Design review of the part built by this model. Coordinates are the model's own, in mm. A direction names the side the tool comes from. Give positions to 0.01 mm unless a question says otherwise; leave off trailing zeros. Loops run counter-clockwise (first coordinate to the right, second up) from the corner with the lowest first, then second, coordinate; pieces in that order, holes last. Notation, with made-up numbers: (55.5, -7.5) -> (103.5, -7.5) arc R29 cw to (103.5, 17.5) -> close; hole circle Ø5 at (65.25, 39.25). An arc over 180 degrees is marked (long way). Answer as CSV lines item,"result".
from build123d import *

# Parameters (mm, degrees)
SKETCH1_W            = 30
SKETCH1_H            = 9
BOSS_EXTRUDE1_DEPTH  = 6
CUT_EXTRUDE1_DEPTH   = 7
LPATTERN2_COUNT      = 8
LPATTERN2_PITCH      = 2
LPATTERN2_COL_COUNT  = 8
LPATTERN2_COL_PITCH  = 2
M3_CLEARANCE_HOLE1_D = 3.2
FILLET1_R            = 5


with BuildPart() as part:
    # Sketch1 → Boss-Extrude1 (new body)
    with BuildSketch(Plane(origin=(0, 0, 0), x_dir=(1, 0, 0), z_dir=(0, 1, 0))):
        with Locations((15, 4.5)):
            Rectangle(SKETCH1_W, SKETCH1_H)
    extrude(amount=BOSS_EXTRUDE1_DEPTH)

    # Sketch2 → Cut-Extrude1 (cut, through all)
    with BuildSketch(Plane(origin=(0, 6, 0), x_dir=(1, 0, 0), z_dir=(0, 1, 0))):
        Polygon((14.41183651, 9), (15.58816349, 9), (15.41183651, 8), (14.58816349, 8), align=None)
    cut_extrude1 = extrude(amount=-CUT_EXTRUDE1_DEPTH, mode=Mode.SUBTRACT)

    # LPattern2: Cut-Extrude1 ×8
    with Locations(*[(-i * LPATTERN2_PITCH, 0, 0) for i in range(1, LPATTERN2_COUNT)]):
        add(cut_extrude1, mode=Mode.SUBTRACT)

    # LPattern2 col: Cut-Extrude1 ×8
    with Locations(*[(i * LPATTERN2_COL_PITCH, 0, 0) for i in range(1, LPATTERN2_COL_COUNT)]):
        add(cut_extrude1, mode=Mode.SUBTRACT)

    # M3 Clearance Hole1 (through all)
    with Locations(Plane(origin=(0, 6, 0), x_dir=(1, 0, 0), z_dir=(0, 1, 0))):
        with Locations((5, 5), (25, 5)):
            Hole(M3_CLEARANCE_HOLE1_D / 2)

    # Fillet1
    fillet1_edges = [part.edges().sort_by_distance(p)[0] for p in [
        (30, 3, 0),
        (0, 3, 0),
    ]]
    fillet(fillet1_edges, radius=FILLET1_R)


solid = part.part
Q1. We need section B-B, the plane z = -3. State the section outline as (x, y) points, and give its area (3 significant figures).
Filled sheet:
outline,"(0.42, 0) -> (29.58, 0) -> (29.58, 6) -> (0.42, 6) -> close"
area,"175 mm^2"
Q2. We need section A-A, the plane y = 4. State how many separate pieces and enclosed holes the cut face has, and give its area (3 significant figures).
Filled sheet:
separate pieces,"1"
enclosed holes,"2"
area,"228 mm^2"
Q3. For faces 1 (the flat face through (14, 3, -9)), 2 (the flat face through (16.5, 3, -8.5)), list the 3-axis set-ups (+Z, -Z, +X, -X, +Y, -Y) from which the entire face can be reached by the end or side of a thin tool; tool diameter is ignored.
Filled sheet:
face 1,"-Z, +X, -X, +Y, -Y"
face 2,"-Z, +Y, -Y"
Q4. Clearance check with flat-ended pins moving along their axes: pin 1 Ø3 at (x, z) = (5, -5) entering from -Y; pin 2 Ø0.7 at (x, y) = (27, 3.5) entering from -Z. State where each tip first meets the part, or that it passes through.
Filled sheet:
pin 1,"passes through"
pin 2,"stops at z = -8"
Q5. To check wall thickness, follow probe 1 along Z at (x, y) = (5, 4.65); probe 2 along X at (y, z) = (5.5, -3); probe 3 along X at (y, z) = (2.5, -3.25). State the ranges of each line that lie inside material, in increasing order. Write a range as from..to.
Filled sheet:
probe 1,"z = -8..-6.6, -3.4..0"
probe 2,"x = 0.42..29.58"
probe 3,"x = 0.32..29.68"
Q6. The part is to be moulded in two halves that separate along X. For faces 3 (the flat face through (29, 3, -8)), 4 (the flat face through (28, 3, -9)), 5 (the flat face through (7, 3, -8)), say which applies: pulls with the +X half, pulls with the -X half, needs draft (parallel to the pull), parting line crosses it, or undercut.
Filled sheet:
face 3,"undercut"
face 4,"needs draft"
face 5,"undercut"
